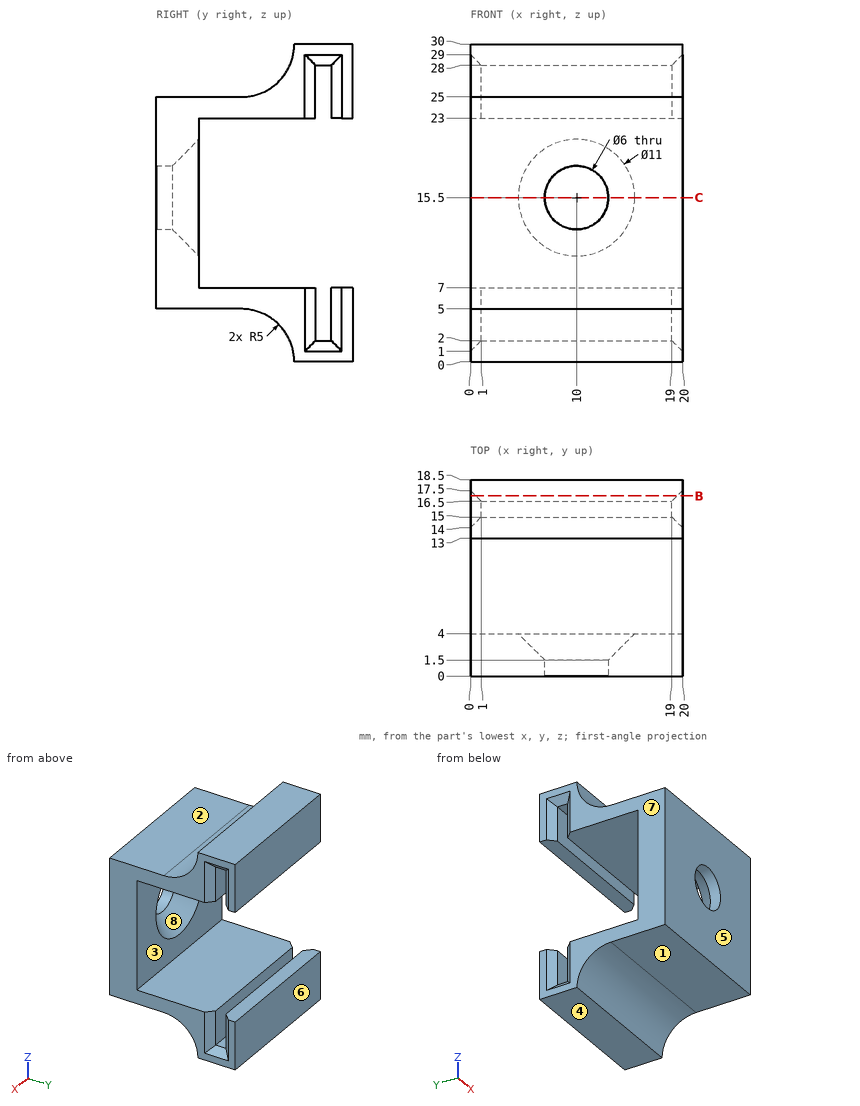
Could you check a few things on this drawing? It's one solid part, dimensions in mm from its lowest x, y, z. A direction names the side the tool comes from. Coordinates: 2 decimals unless noted, no trailing zeros. Order: outer loops, then holes, each group sorted by start corner. A loop starts at its lowest first (then second) coordinate and runs counter-clockwise, first axis right, second up. Notation, with made-up numbers: M 52,29 L 104,29 A33 ccw 104,67 Z; hole C -4.5,-33 d4. An arc over 180 degrees is marked long. Answer as a JSON object with one key per item and string values. Group by question number.
(1) Suppose I cut it at C-C, the plane z = 15.5. Please give me the cut outline in (x, y).
(2) If we mould it in two halves opening along X, with no side actions, what happens to the marked faces 6, 7 and 8? For each: released by +X, released by -X, zero draft, split by the parting line, or undercut.
(3) For pin 1 (5 mm diameter, centred on x = 9, y = 3.5, fed in from -Z); pin 2 (4 mm diameter, centred on x = 6, y = 5.5, fed in from +Z); pin 3 (9.5 mm diameter, centred on x = 10, z = 15.5, fed in from +Y), each with a flat end and sliding along its axis, tell me the tip position at first contact or that it passes through.
(4) I need wall thicknesses on probe 1 along X at (y, z) = (0.9, 15.5); probe 2 along Z at (x, y) = (15.25, 15.25); probe 3 along Z at (x, y) = (10, 0.9). Which ranges of each line are inside material? Lowest first, please.
(5) Suppose I cut it at B-B, the plane y = 17. Please give me the cut outline in (x, z).
(6) Which directions (+Z, -Z, +X, -X, +Y, -Y) give clear straight access to the entire face, cutting with the end or side of a thin tool? Please do the marked faces 1, 2, 3, 4 and 5.
Values found:
{
 "1": {"outline": "M 0,0 L 7,0 L 7,1.5 L 4.5,4 L 0,4 Z; M 13,0 L 20,0 L 20,4 L 15.5,4 L 13,1.5 Z"},
 "2": {"face 6": "zero draft", "face 7": "released by -X", "face 8": "undercut"},
 "3": {"pin 1": "stops at z = 5", "pin 2": "stops at z = 25", "pin 3": "stops at y = 3.25"},
 "4": {"probe 1": "x = 0 to 7, 13 to 20", "probe 2": "z = 0 to 2, 28 to 30", "probe 3": "z = 5 to 12.5, 18.5 to 25"},
 "5": {"outline": "M 0,0 L 20,0 L 20,1 L 19.5,1.5 L 19.5,7 L 0.5,7 L 0.5,1.5 L 0,1 Z; M 0,29 L 0.5,28.5 L 0.5,23 L 19.5,23 L 19.5,28.5 L 20,29 L 20,30 L 0,30 Z"},
 "6": {"face 1": "-Z, +X, -X, -Y", "face 2": "+Z, +X, -X, -Y", "face 3": "+X, -X, +Y", "face 4": "-Z, +X, -X, +Y, -Y", "face 5": "+Z, -Z, +X, -X, -Y"}
}
